Geometry check sheet. Reference: the model listing, model coordinates, mm. A direction names the side the tool comes from. Give positions to 0.01 mm unless a question says otherwise; leave off trailing zeros. Loops run counter-clockwise (first coordinate to the right, second up) from the corner with the lowest first, then second, coordinate; pieces in that order, holes last. Notation, with made-up numbers: (-0.75, -27) -> (53.25, -27) arc R22 ccw to (53.25, -4) -> close; hole circle Ø4 at (30.25, 38). An arc over 180 degrees is marked (long way). One line per item, written item: value. Start each with the question number.
(1) Tool access check on faces 4 (the face through (69.5, -1, 12)), 5 (the face through (44, -1, 50)). Record the directions out of +Z, -Z, +X, -X, +Y, -Y that give a thin tool (end or side, any length) a straight path to the whole face; none if there is none.
(2) Sectioned sample at C-C, the plane z = -23.1. Record the cut outline in (x, y).
(3) Sectioned sample at A-A, the plane x = 73. Record the cut outline in (y, z), then the cut area to 3 significant figures.
(4) Scan lines: line 1 along Z through (x, y) = (70, -1.15); line 2 along X through (y, z) = (-0.75, -23.1); line 3 along Z through (x, y) = (21, -0.65). Record each from-to range of solid material in increasing order. Write a range as from..to.
(5) Gauge pin test, flat end, axial feed: pin 1 Ø3.5 at (x, z) = (21, -35.1) entering from -Y. Record the tip position at first contact, or that the pin passes through.
(6) Draft check along X on faces 1 (the face through (120, -1, 1)), 2 (the face through (30.5, -1, 12)), 3 (the face through (44, -1, -50)). Enter one of: pulls with the +X half, pulls with the -X half, needs draft (parallel to the pull), parting line crosses it, or undercut.
(7) Sectioned sample at B-B, the plane x = 21. Record the cut outline in (y, z), then the cut area to 3 significant figures.
from build123d import *

# Parameters (mm, degrees)
SKETCH1_W                     = 150
SKETCH1_H                     = 100
BASEPLATE_DEPTH               = 3
F_6_CLEARANCE_HOLE1_D         = 3.7973
SKETCH4_W                     = 11
SKETCH4_H                     = 3
BASETABHOLE_DEPTH             = 131.034610777
BASETABHOLEPATTERN_COUNT      = 2
BASETABHOLEPATTERN_PITCH      = 50
BASETABHOLEPATTERN_COUNT_DIR2 = 2
BASETABHOLEPATTERN_PITCH_DIR2 = 23


with BuildPart() as part:
    # Sketch1 → BasePlate (new body)
    with BuildSketch(Plane(origin=(0, 0, 0), x_dir=(1, 0, 0), z_dir=(0, 1, 0))):
        with Locations((45, 0)):
            Rectangle(SKETCH1_W, SKETCH1_H)
    extrude(amount=-BASEPLATE_DEPTH)

    # #6 Clearance Hole1 (through all)
    with Locations(Plane(origin=(0, 0, 0), x_dir=(1, 0, 0), z_dir=(0, 1, 0))):
        with Locations((-21, 23.1), (21, 23.1), (21, 35.1), (-21, 35.1)):
            Hole(F_6_CLEARANCE_HOLE1_D / 2)

    # Sketch4 → BaseTabHole (cut, through all)
    with BuildSketch(Plane(origin=(0, 0, 0), x_dir=(1, 0, 0), z_dir=(0, 1, 0))):
        with Locations((25, 11.5)):
            Rectangle(SKETCH4_W, SKETCH4_H)
    basetabhole = extrude(amount=-BASETABHOLE_DEPTH, mode=Mode.SUBTRACT)

    # BaseTabHolePattern: BaseTabHole 2 × 2
    with Locations(*[(i * BASETABHOLEPATTERN_PITCH, 0, j * BASETABHOLEPATTERN_PITCH_DIR2) for i in range(BASETABHOLEPATTERN_COUNT) for j in range(BASETABHOLEPATTERN_COUNT_DIR2) if (i, j) != (0, 0)]):
        add(basetabhole, mode=Mode.SUBTRACT)


solid = part.part
Calculated:
1. face 4: +Y, -Y
1. face 5: +Z, +X, -X, +Y, -Y
2. outline: (-30, -3) -> (-22.9, -3) -> (-22.9, 0) -> (-30, 0) -> close; (-19.1, -3) -> (19.1, -3) -> (19.1, 0) -> (-19.1, 0) -> close; (22.9, -3) -> (120, -3) -> (120, 0) -> (22.9, 0) -> close
3. outline: (-3, -50) -> (0, -50) -> (0, -13) -> (-3, -13) -> close; (-3, -10) -> (0, -10) -> (0, 10) -> (-3, 10) -> close; (-3, 13) -> (0, 13) -> (0, 50) -> (-3, 50) -> close
3. area: 282 mm2
4. line 1: z = -50..-13, -10..10, 13..50
4. line 2: x = -30..-22.9, -19.1..19.1, 22.9..120
4. line 3: z = -50..-37, -33.2..-25, -21.2..-13, -10..10, 13..50
5. pin 1: passes through
6. face 1: pulls with the +X half
6. face 2: undercut
6. face 3: needs draft
7. outline: (-3, -50) -> (0, -50) -> (0, -37) -> (-3, -37) -> close; (-3, -33.2) -> (0, -33.2) -> (0, -25) -> (-3, -25) -> close; (-3, -21.2) -> (0, -21.2) -> (0, -13) -> (-3, -13) -> close; (-3, -10) -> (0, -10) -> (0, 10) -> (-3, 10) -> close; (-3, 13) -> (0, 13) -> (0, 50) -> (-3, 50) -> close
7. area: 259 mm2
